Read the model definition and answer for the solid it produces. Units are mm, in the model's axes. Coordinates: 2 decimals unless noted, no trailing zeros. Loops run counter-clockwise (first coordinate to the right, second up) from the corner with the lowest first, then second, coordinate; pieces in that order, holes last. Notation, with made-up numbers: M 51.25,-9.5 L 97.25,-9.5 A17 cw 97.25,-0.5 Z; hole C 85.25,20 d2. An arc over 180 degrees is marked long. One line per item, written item: value. Start each with the question number.
```python
from build123d import *

# Parameters (mm, degrees)
SKETCH1_R                 = 1.01
SKETCH1_R_2               = 3.5
BOSS_EXTRUDE2_DEPTH       = 3.175
F_2_CLEARANCE_HOLE1_D     = 2.4384
F_2_CLEARANCE_HOLE1_DEPTH = 3.302
F_2_CLEARANCE_HOLE1_TIP   = 0.732569267
M2_5X0_45_TAPPED_HOLE1_D  = 2.05


with BuildPart() as part:
    # Sketch1 → Boss-Extrude2 (new body)
    with BuildSketch(Plane.XY):
        with BuildLine():
            Line((0, 0), (37, 0))
            Line((37, 0), (37, 7.50213794))
            ThreePointArc((37, 7.50213794), (30.666699296, 14), (37, 20.49786206))
            Line((37, 20.49786206), (37, 32))
            Line((37, 32), (0, 32))
            Line((0, 32), (0, 0))
        make_face()
        with Locations((25.169778966, 21.933400182)):
            Circle(SKETCH1_R, mode=Mode.SUBTRACT)
        with Locations((16, 16)):
            Circle(SKETCH1_R_2, mode=Mode.SUBTRACT)
    extrude(amount=BOSS_EXTRUDE2_DEPTH)

    # #2 Clearance Hole1
    with Locations(Plane.XY.offset(3.175)):
        with Locations((3, 29), (3, 3), (34, 29), (26, 3)):
            Hole(F_2_CLEARANCE_HOLE1_D / 2, depth=F_2_CLEARANCE_HOLE1_DEPTH)
            with Locations((0, 0, -(F_2_CLEARANCE_HOLE1_DEPTH + F_2_CLEARANCE_HOLE1_TIP / 2))):  # 118° drill point
                Cone(0, F_2_CLEARANCE_HOLE1_D / 2, F_2_CLEARANCE_HOLE1_TIP, mode=Mode.SUBTRACT)

    # M2.5x0.45 Tapped Hole1 (through all)
    with Locations(Plane.XY.offset(3.175)):
        with Locations((8, 16), (12, 22.92820323), (20, 22.92820323), (24, 16), (20, 9.07179677), (12, 9.07179677), (16, 16)):
            Hole(M2_5X0_45_TAPPED_HOLE1_D / 2)


solid = part.part
```
1) For a pull along X with two mould halves and no side action, classify faces 1 (the face through (30.67, 13.86, 1.57)), 2 (the face through (24.76, 16.69, 1.57)), 3 (the face through (2.437, 1.918, 1.565)), 4 (the face through (19, 32, 2)) as released by +X, released by -X, zero draft, split by the parting line, or undercut.
2) Section A-A (y = 3) is taken. Determine the outline of the cut face in (x, z) (3 decimals).
3) Section B-B (x = 16) is taken. Determine the outline of the cut face in (y, z) (3 decimals).
4) Consider line 1 along Y through (x, z) = (12, 1.25); line 2 along Y through (x, z) = (24, 2.2) (3 decimals); line 3 along Y through (x, z) = (3, 2.25). Determine where each line is inside the solid, lowest interval first.
5) Section C-C (x = 20) is taken. Determine the outline of the cut face in (y, z) (3 decimals), then the cut area to 3 significant figures.
6) A flat-ended cylindrical pin translates along its axis: pin 1 (1.6 mm diameter, centred on x = 12, y = 22.93, fed in from +Z). Find the tip coordinate at first contact, or state that the pin passes through.
7) Section D-D (y = 18.5) is taken. Determine the outline of the cut face in (x, z) (3 decimals), then the cut area to 3 significant figures.
Results found:
1. face 1: released by +X
1. face 2: undercut
1. face 3: undercut
1. face 4: zero draft
2. outline: M 0,0 L 1.781,0 L 1.781,3.175 L 0,3.175 Z; M 4.219,0 L 24.781,0 L 24.781,3.175 L 4.219,3.175 Z; M 27.219,0 L 37,0 L 37,3.175 L 27.219,3.175 Z
3. outline: M 0,0 L 12.5,0 L 12.5,3.175 L 0,3.175 Z; M 19.5,0 L 32,0 L 32,3.175 L 19.5,3.175 Z
4. line 1: y = 0 to 8.05, 10.1 to 21.9, 23.95 to 32
4. line 2: y = 0 to 14.975, 17.025 to 32
4. line 3: y = 0 to 1.78, 4.22 to 27.78, 30.22 to 32
5. outline: M 0,0 L 8.047,0 L 8.047,3.175 L 0,3.175 Z; M 10.097,0 L 21.903,0 L 21.903,3.175 L 10.097,3.175 Z; M 23.953,0 L 32,0 L 32,3.175 L 23.953,3.175 Z
5. area: 88.6 mm²
6. pin 1: passes through
7. outline: M 0,0 L 13.551,0 L 13.551,3.175 L 0,3.175 Z; M 18.449,0 L 32.476,0 L 32.476,3.175 L 18.449,3.175 Z
7. area: 87.6 mm²
